Design review of the part built by this model. Coordinates are the model's own, in mm. A direction names the side the tool comes from. Coordinates: 2 decimals unless noted, no trailing zeros. Order: outer loops, then holes, each group sorted by start corner. A loop starts at its lowest first (then second) coordinate and runs counter-clockwise, first axis right, second up. Notation, with made-up numbers: (7.25, 25) -> (11.25, 25) arc R25 ccw to (11.25, 52) -> close; hole circle Ø1 at (28.25, -33.5). An arc over 180 degrees is marked (long way). Write item = value, one per line.
```python
from build123d import *

# Parameters (mm, degrees)
SKETCH1_R           = 4
BOSS_EXTRUDE1_DEPTH = 1.5


with BuildPart() as part:
    # Sketch1 → Boss-Extrude1 (new, symmetric)
    with BuildSketch(Plane(origin=(0, 0, 0), x_dir=(1, 0, 0), z_dir=(0, 1, 0))):
        with BuildLine():
            Line((-10, -8.624404748), (-14.5, -8.624404748))
            ThreePointArc((-14.5, -8.624404748), (-17.681980515, -9.942424233), (-19, -13.124404748))
            Line((-19, -13.124404748), (-19, -14.124404748))
            ThreePointArc((-19, -14.124404748), (-17.681980515, -17.306385264), (-14.5, -18.624404748))
            Line((-14.5, -18.624404748), (4.5, -18.624404748))
            ThreePointArc((4.5, -18.624404748), (7.681980515, -19.942424233), (9, -23.124404748))
            Line((9, -23.124404748), (9, -24.124404748))
            ThreePointArc((9, -24.124404748), (10.318019485, -27.306385264), (13.5, -28.624404748))
            Line((13.5, -28.624404748), (14.5, -28.624404748))
            ThreePointArc((14.5, -28.624404748), (17.681980515, -27.306385264), (19, -24.124404748))
            Line((19, -24.124404748), (19, -13.124404748))
            ThreePointArc((19, -13.124404748), (17.681980515, -9.942424233), (14.5, -8.624404748))
            Line((14.5, -8.624404748), (10, -8.624404748))
            ThreePointArc((10, -8.624404748), (12.023420987, -16.074878268), (6.509119733, -10.671520993))
            ThreePointArc((6.509119733, -10.671520993), (0, -12.5), (-6.509119733, -10.671520993))
            ThreePointArc((-6.509119733, -10.671520993), (-12.023420987, -16.074878268), (-10, -8.624404748))
        make_face()
        with Locations(Location((14, -23.124404748, 0), (0, 0, 270))):
            Circle(SKETCH1_R, mode=Mode.SUBTRACT)
    extrude(amount=BOSS_EXTRUDE1_DEPTH, both=True)


solid = part.part
```
(1) Insertion check: pin 1 (1.5 mm diameter, centred on x = -1, y = -0.5, fed in from -Z); pin 2 (9 mm diameter, centred on x = 10, z = 12.62, fed in from -Y); pin 3 (1.5 mm diameter, centred on x = 7, y = -1, fed in from -Z); pin 4 (6 mm diameter, centred on x = -13, z = 24.5, fed in from +Y). Each pin has a flat end and moves straight along its axis. Give the tip position at first contact, or say it passes through.
Report:
pin_1 = 12.38
pin_2 = -1.5
pin_3 = 10.67
pin_4 = through
(2) We need section C-C (x = -13). Write out the cut boundary in (y, z), and give its area (3 significant figures).
Report:
outline = (-1.5, 8.62) -> (1.5, 8.62) -> (1.5, 9.98) -> (-1.5, 9.98) -> close; (-1.5, 15.27) -> (1.5, 15.27) -> (1.5, 18.62) -> (-1.5, 18.62) -> close
area = 14.1 mm²
(3) We need section B-B (z = 19.5). Write out the cut boundary in (x, y), and give its area (3 significant figures).
Report:
outline = (7.17, -1.5) -> (12.31, -1.5) -> (12.31, 1.5) -> (7.17, 1.5) -> close; (15.69, -1.5) -> (19, -1.5) -> (19, 1.5) -> (15.69, 1.5) -> close
area = 25.3 mm²
(4) We need section D-D (x = 0.5). Write out the cut boundary in (y, z), and give its area (3 significant figures).
Report:
outline = (-1.5, 12.49) -> (1.5, 12.49) -> (1.5, 18.62) -> (-1.5, 18.62) -> close
area = 18.4 mm²
(5) For L1, parallel to X at y = -0.45, z = 23; L2, parallel to X at y = 0.9, z = 14.5; L3, parallel to X at y = 1.15, z = 13, list the stretches that pass through material, from the lowest coordinate up.
Report:
L1 = 9 to 10, 18 to 19
L2 = -18.98 to -13.53, -6.47 to 6.47, 13.53 to 19
L3 = -19 to -13.98, -6.02 to 6.02, 13.98 to 19
(6) The part is to be moulded in two halves that separate along X. For faces 1 (the cylindrical face through (12.148, 0.021, 15.999)), 2 (the flat face through (3, -1.5, 16)), 3 (the cylindrical face through (7.65, 0.02, 19.91)), 4 (the cylindrical face through (16.703, -0.021, 20.176)), say which applies: released by +X, released by -X, zero draft, split by the parting line, or undercut.
Report:
face_1 = undercut
face_2 = zero draft
face_3 = released by -X
face_4 = undercut
(7) For faces 5 (the flat face through (9, 0, 23.6)), 6 (the flat face through (19, 0, 19)), list the 3-axis set-ups (+Z, -Z, +X, -X, +Y, -Y) from which the entire face can be reached by the end or side of a thin tool; tool diameter is ignored.
Report:
face_5 = +Z, -X, +Y, -Y
face_6 = +Z, -Z, +X, +Y, -Y
(8) We need section A-A (y = 0.35). Write out the cut boundary in (x, z).
Report:
outline = (-19, 13.12) arc R4.5 ccw to (-14.5, 8.62) -> (-10, 8.62) arc R4 cw (long way) to (-6.51, 10.67) arc R12.5 cw to (6.51, 10.67) arc R4 cw (long way) to (10, 8.62) -> (14.5, 8.62) arc R4.5 ccw to (19, 13.12) -> (19, 24.12) arc R4.5 ccw to (14.5, 28.62) -> (13.5, 28.62) arc R4.5 ccw to (9, 24.12) -> (9, 23.12) arc R4.5 cw to (4.5, 18.62) -> (-14.5, 18.62) arc R4.5 ccw to (-19, 14.12) -> close; hole circle Ø8 at (14, 23.12)
